Geometry check sheet. Reference: drawing and pictorial views, mm from the part's lowest x, y, z. Give positions to 0.01 mm unless a question says otherwise; leave off trailing zeros. Write each loop counter-clockwise with the first axis right and the second up, starting at its lowest first coordinate (ties: lowest second). Pieces come first, ordered by that corner, then holes. Notation, with made-up numbers: M 10,-26 L 21,-26 A35 cw 21,8 Z; hole C 44.5,70 d6. An arc over 180 degrees is marked long. Write item = value, one per line. Start each with the question number.
1) Cross-section at A-A, the plane x = 187.5. Record the cut outline in (y, z).
2) Cross-section at B-B, the plane z = 16.5. Give the number of separate pieces and of enclosed holes in the cut face, plus the area to 3 significant figures.
3) Cross-section at D-D, the plane z = 56. Record the cut outline in (x, y) (3 decimals).
4) Scan lines: line 1 along X through (y, z) = (32.5, 19.5); line 2 along X through (y, z) = (31.5, 16); line 3 along Y through (x, z) = (31, 45). Record each from-to range of solid material in increasing order. Write a range as [from, to].
5) Go/stop test with flat-tipped pins: pin 1 (12 mm diameter, centred on x = 49.5, z = 66.5, fed in from +Y); pin 2 (4 mm diameter, centred on y = 47, z = 34.5, fed in from -X); pin 3 (4 mm diameter, centred on y = 40.5, z = 43.5, fed in from -X). Record where each tip stops, or that it passes through.
6) Cross-section at C-C, the plane y = 59. Record the cut outline in (x, z).
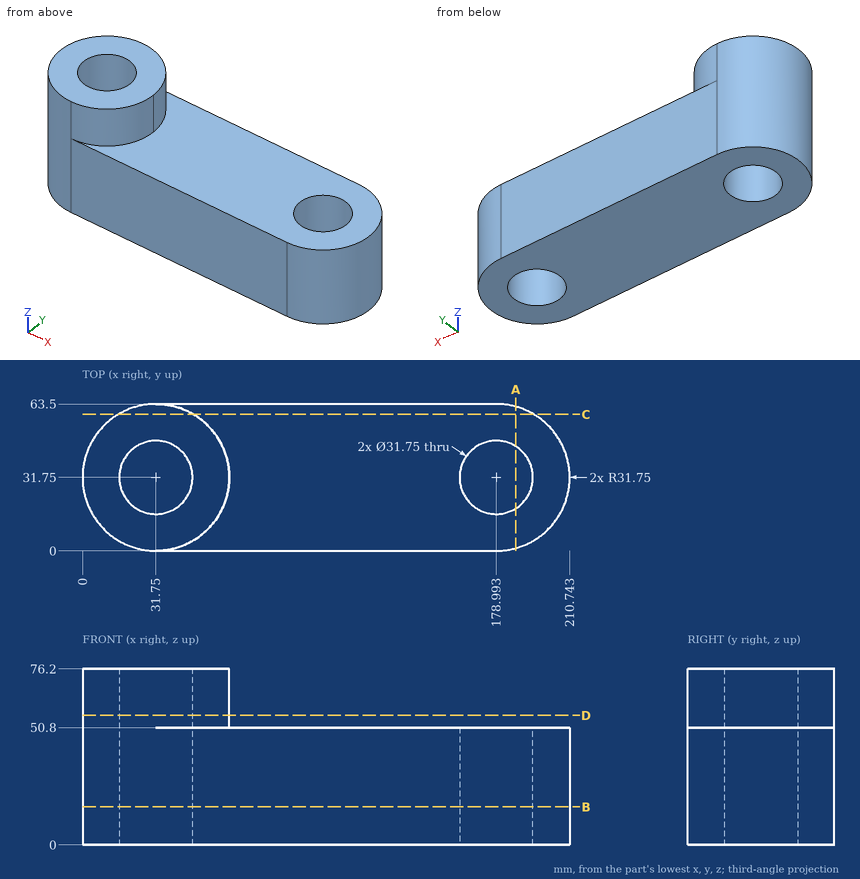
Reply:
q1.outline = M 1.16,0 L 18.35,0 L 18.35,50.8 L 1.16,50.8 Z; M 45.15,0 L 62.34,0 L 62.34,50.8 L 45.15,50.8 Z
q2.separate_pieces = 1
q2.enclosed_holes = 2
q2.area = 10,900 mm2
q3.outline = M 31.75,0 A31.75 ccw 63.5,31.75 A31.75 ccw long Z; hole C 31.75,31.75 d31.75
q4.line_1 = [0.01, 15.89], [47.61, 163.14], [194.85, 210.73]
q4.line_2 = [0, 15.88], [47.62, 163.12], [194.87, 210.74]
q4.line_3 = [0.01, 15.89], [47.61, 63.49]
q5.pin_1 = 61.25
q5.pin_2 = 2.9
q5.pin_3 = 0.73
q6.outline = M 15.46,0 L 195.29,0 L 195.29,50.8 L 48.04,50.8 L 48.04,76.2 L 15.46,76.2 Z
